from build123d import *

# Parameters (mm, degrees)
PAD_DEPTH            = 65
SKETCH001_W          = 25
SKETCH001_H          = 40
POCKET_DEPTH         = 50.001
SKETCH002_W          = 20
SKETCH002_H          = 40
POCKET001_DEPTH      = 50.001
SKETCH003_W          = 50
SKETCH003_H          = 35
POCKET002_DEPTH      = 25.001
POCKET002_DEPTH_BACK = -25.001
POCKET003_DEPTH      = 15.001
PAD001_DEPTH         = 5
POCKET004_DEPTH      = 50.001


with BuildPart() as part:
    # Sketch → Pad (new body)
    with BuildSketch(Plane.XZ):
        with BuildLine():
            Line((-25, 80), (-25, 0))
            Line((-25, 0), (25, 0))
            Line((25, 0), (25, 80))
            ThreePointArc((25, 80), (0, 105), (-25, 80))
        make_face()
    extrude(amount=-PAD_DEPTH)

    # Sketch001 (on Face3 of Pad) → Pocket (cut, through all)
    with BuildSketch(Plane(origin=(25, 0, 0), x_dir=(0, 0, 1), z_dir=(1, 0, 0))):
        with Locations((12.5, -45)):
            Rectangle(SKETCH001_W, SKETCH001_H)
    extrude(amount=-POCKET_DEPTH, mode=Mode.SUBTRACT)

    # Sketch002 (on Face8 of Pocket) → Pocket001 (cut, through all)
    with BuildSketch(Plane(origin=(25, 0, 0), x_dir=(0, 0, 1), z_dir=(1, 0, 0))):
        with Locations((60, -45)):
            Rectangle(SKETCH002_W, SKETCH002_H)
    extrude(amount=-POCKET001_DEPTH, mode=Mode.SUBTRACT)

    # Sketch003 → Pocket002 (cut, two sides)
    with BuildSketch(Plane.YZ) as pocket002_sk:
        with Locations((40, 87.5)):
            Rectangle(SKETCH003_W, SKETCH003_H)
    extrude(amount=-POCKET002_DEPTH, mode=Mode.SUBTRACT)
    extrude(pocket002_sk.sketch, amount=-POCKET002_DEPTH_BACK, mode=Mode.SUBTRACT)

    # Sketch004 (on Face10 of Pocket002) → Pocket003 (cut, through all)
    with BuildSketch(Plane(origin=(0, 15, 0), x_dir=(1, 0, 0), z_dir=(0, 1, 0))):
        with BuildLine():
            ThreePointArc((-15, -80), (0, -95), (15, -80))
            Line((15, -80), (-15, -80))
        make_face()
    extrude(amount=-POCKET003_DEPTH, mode=Mode.SUBTRACT)

    # Sketch005 → Pad001 (join, symmetric)
    with BuildSketch(Plane.YZ):
        Polygon((25, 70), (25, 50), (45, 50), align=None)
    extrude(amount=PAD001_DEPTH, both=True)

    # Sketch006 (on Face7 of Pad001) → Pocket004 (cut, through all)
    with BuildSketch(Plane(origin=(0, 0, 50), x_dir=(-1, 0, 0), z_dir=(0, 0, 1))):
        with BuildLine():
            ThreePointArc((15, -65), (0, -50), (-15, -65))
            Line((-15, -65), (15, -65))
        make_face()
    extrude(amount=-POCKET004_DEPTH, mode=Mode.SUBTRACT)


solid = part.part
Design review of the part built by this model. Coordinates are the model's own, in mm. A direction names the side the tool comes from. Round coordinates to 2 decimals unless told otherwise and drop trailing zeros. Loops run counter-clockwise (first coordinate to the right, second up) from the corner with the lowest first, then second, coordinate; pieces in that order, holes last. Notation, with made-up numbers: M 14,-8 L 31,-8 A15 cw 31,18 Z; hole C -12,-33.75 d7. An arc over 180 degrees is marked long. Answer as a JSON object with one key per item and string values.
Item 1: Wall thickness on L1, parallel to Y at x = -19.5, z = 68.5; L2, parallel to Z at x = 1.5, y = 21; L3, parallel to X at y = 31.5, z = 52.5: over which ranges is each line inside the solid? List them lowest first. Write a range as from..to.
Answer sheet:
{"L1": "y = 0..25", "L2": "z = 0..70", "L3": "x = -5..5"}
Item 2: We need section A-A on x = 0. Give the boundary of the cut face in (y, z).
Answer sheet:
{"outline": "M 0,0 L 25,0 L 25,25 L 50,25 L 50,50 L 45,50 L 25,70 L 15,70 L 15,80 L 0,80 Z; M 0,95 L 15,95 L 15,105 L 0,105 Z"}
Item 3: The part is to be moulded in two halves that separate along X. For faces 6 (the flat face through (-25, 25, 41)), 7 (the flat face through (0, 8, 80)), 8 (the flat face through (20, 65, 38)), say which applies: pulls with the +X half, pulls with the -X half, needs draft (parallel to the pull), parting line crosses it, or undercut.
Answer sheet:
{"face 6": "pulls with the -X half", "face 7": "undercut", "face 8": "needs draft"}
Item 4: Machinability: for faces 1 (the flat face through (0.4, 45.3, 50)), 2 (the flat face through (15, 25, 60)), 3 (the flat face through (0, 41, 25)), 4 (the flat face through (-5, 30, 56)), 5 (the flat face through (0, 15, 79)), which of the approach directions +Z, -Z, +X, -X, +Y, -Y give a long, thin tool a straight path to every point of the face, cutting with its end or side? Answer none if there is none.
Answer sheet:
{"face 1": "+Z, +Y", "face 2": "+Z, +X, +Y", "face 3": "-Z, +X, -X, +Y", "face 4": "+Z, -X, +Y", "face 5": "+Z, +X, -X, +Y"}
Item 5: We need section D-D on y = 10.5. Give the boundary of the cut face in (x, z).
Answer sheet:
{"outline": "M -25,0 L 25,0 L 25,80 A25 ccw -25,80 Z; hole M -15,80 L 15,80 A15 ccw Z"}
Item 6: Clearance check with flat-ended pins moving along their axes: P1, Ø20, axis at x = -6, z = 7, coming from the +Y side; P2, Ø10, axis at x = 8, y = 53.5, coming from the -Z side; P3, Ø16, axis at y = 40, z = 63, coming from the -X side; P4, Ø10, axis at x = 4.5, y = 58, coming from the -Z side. State where each tip first meets the part, or that it passes through.
Answer sheet:
{"P1": "stops at y = 25", "P2": "stops at z = 25", "P3": "stops at x = -5", "P4": "passes through"}
Item 7: We need section C-C on z = 86.5. Give the boundary of the cut face in (x, y), and give its area (3 significant figures).
Answer sheet:
{"outline": "M -24.14,0 L -13.52,0 L -13.52,15 L -24.14,15 Z; M 13.52,0 L 24.14,0 L 24.14,15 L 13.52,15 Z", "area": "319 mm^2"}
Item 8: We need section B-B on y = 57.5. Give the boundary of the cut face in (x, z).
Answer sheet:
{"outline": "M -25,25 L -12.99,25 L -12.99,50 L -25,50 Z; M 12.99,25 L 25,25 L 25,50 L 12.99,50 Z"}
